Job drawing, mm, ordinate dimensions from the low corner. One solid piece. A direction names the side the tool comes from. Coordinates: 2 decimals unless noted, no trailing zeros. Order: outer loops, then holes, each group sorted by start corner. A loop starts at its lowest first (then second) coordinate and runs counter-clockwise, first axis right, second up. Notation, with made-up numbers: (25, -23.5) - (52, -23.5) arc R29 cw to (52, 11.5) - close; hole circle Ø2 at (-30, 62). An arc over 180 degrees is marked (long way). Use a Markdown table: item, result. Add a question column.
1) Two-plate mould, pull along Z, no slides. Class the marked faces 1, 2, 3 and 4: +Z half, -Z half, draft (parallel to the pull), parting line (faces both ways), or undercut.
2) Tool access for the marked faces 5, 6 and 7: list every direction of +Z, -Z, +X, -X, +Y, -Y with a clear straight run to the whole face (end or side of a thin tool).
3) Wall check: L1, parallel to Y at x = 7.75, z = 2.05; L2, parallel to Y at x = 7.75, z = 4.3; L3, parallel to Y at x = 7.25, z = 1.5. Give the ranges that are in metal, low to high. Write a range as [from, to].
4) Saw through at D-D on y = 13.5. List the corners of the cut face in (x, z), then the cut area to 3 significant figures.
5) Saw through at A-A on x = 7.75. Count the separate pieces of the cut face and the enclosed holes in it, then the cut area to 3 significant figures.
6) Saw through at C-C on y = 3.5. List the corners of the cut face in (x, z).
7) Drop flat-ended pins along their axis: P1, Ø1, axis at x = 3.5, y = 2, coming from the +Z side; P2, Ø5, axis at x = 10.5, y = 3.5, coming from the +Z side; P3, Ø2.5, axis at y = 3.5, z = 7.75, coming from the -X side. Give the stop position or say it passes through.
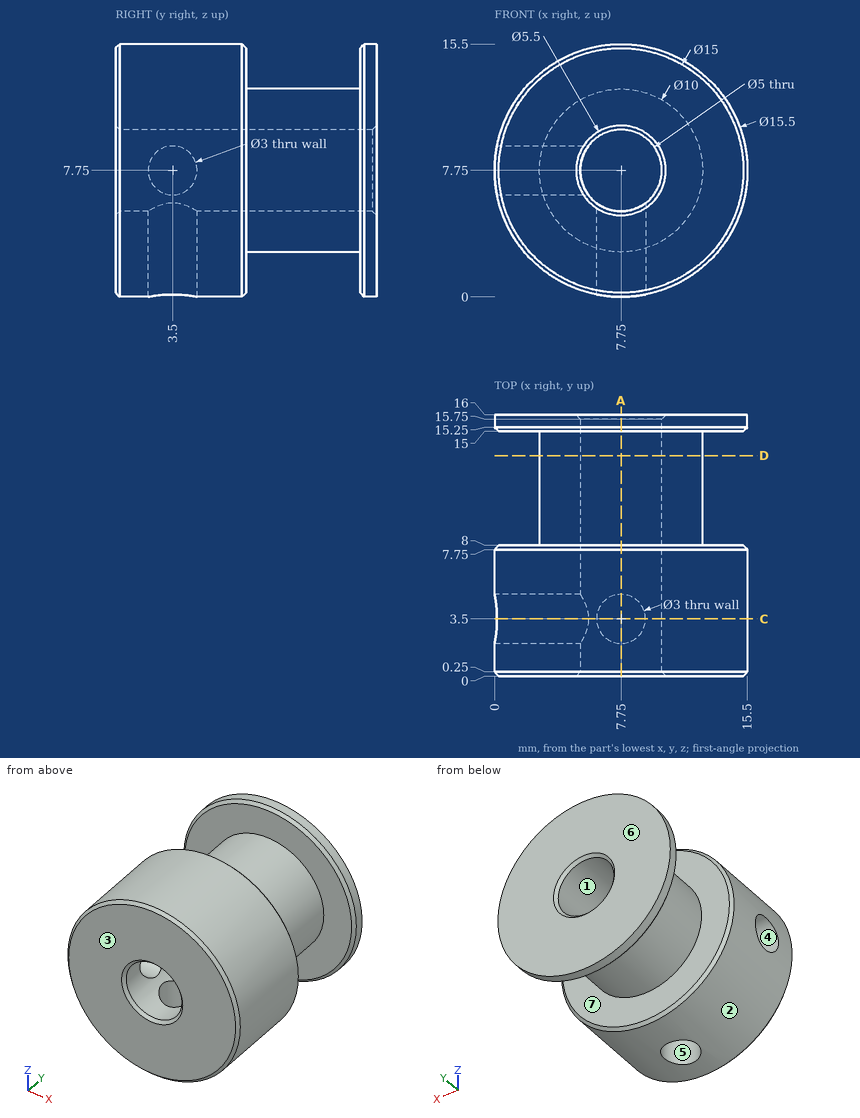
Results are:
| question | item | result |
|---|---|---|
| 1 | face 1 | undercut |
| 1 | face 2 | parting line |
| 1 | face 3 | draft |
| 1 | face 4 | undercut |
| 2 | face 5 | -Z |
| 2 | face 6 | +Z, -Z, +X, -X, +Y |
| 2 | face 7 | none |
| 3 | L1 | [0, 2], [5, 8], [15, 16] |
| 3 | L2 | [0, 2], [5, 16] |
| 3 | L3 | [0, 2.09], [4.91, 8], [15, 16] |
| 4 | outline | circle Ø10 at (7.75, 7.75); hole circle Ø5 at (7.75, 7.75) |
| 4 | area | 58.9 mm2 |
| 5 | separate pieces | 3 |
| 5 | enclosed holes | 0 |
| 5 | area | 113 mm2 |
| 6 | outline | (0.15, 6.25) arc R7.75 ccw to (6.25, 0.15) - (6.25, 5.75) arc R2.5 cw to (5.75, 6.25) - close; (0.15, 9.25) - (5.75, 9.25) arc R2.5 cw (long way) to (9.25, 5.75) - (9.25, 0.15) arc R7.75 ccw (long way) to start |
| 7 | P1 | z = 14.53 |
| 7 | P2 | z = 15.5 |
| 7 | P3 | x = 9.92 |
